Input: part model. Units: mm. Frame: model coordinates. Face numbers are marked on the shaded views. A direction names the side the tool comes from. Round coordinates to 2 decimals unless told otherwise and drop trailing zeros. Loops run counter-clockwise (first coordinate to the right, second up) from the corner with the lowest first, then second, coordinate; pieces in that order, holes last. Notation, with made-up numbers: M 33,16.25 L 81,16.25 A21 cw 81,48.25 Z; hole C -13,9.25 d11. An arc over 180 degrees is marked long. Return JSON: item names as keys, results as strings. Group by question number.
1) Access query for the marked faces 5, 6, 7 and 8. Directions: +Z, -Z, +X, -X, +Y, -Y. A direction counts if a zero-diameter tool reaches every point of the face in a straight line with its end or side. Return the directions, or none.
2) Section C-C (x = 0). Output: boundary loops of the cut face in (y, z).
3) Contact query for flat-ended pins moving along their axis: P1, Ø3.5, axis at x = 11, z = -1, coming from the +Y side; P2, Ø9, axis at x = -3.5, z = -5.5, coming from the +Y side; P3, Ø8, axis at x = 0, y = 0, coming from the -Z side. Output: stop coordinate, or through.
4) Section B-B (z = 3.75). Output: boundary loops of the cut face in (x, y).
5) Section D-D (y = -4.75). Output: boundary loops of the cut face in (x, z), plus the area to 3 significant figures.
6) Mould query, pull axis Y, two halves, no side actions, for the marked faces 1, 2, 3 and 4. Classes: +Y half, -Y half, draft (parallel to the pull), parting line (faces both ways), or undercut.
7) Section A-A (z = -7.75). Output: boundary loops of the cut face in (x, y).
8) Material intervals for line 1 (Y direction, x = 0, z = 2.5); line 2 (X direction, y = -8, z = -2.25); line 3 (X direction, y = 0, z = 4), sorted ascending. Write a range as from..to.
from build123d import *

# Parameters (mm, degrees)
PAD_DEPTH       = 10
SKETCH001_R     = 2.55
POCKET_DEPTH    = 8
CHAMFER_SIZE    = 4
PAD001_DEPTH    = 10
SKETCH003_W     = 13
SKETCH003_H     = 6.844848
POCKET001_DEPTH = 19.501
FILLET_R        = 2


with BuildPart() as part:
    # Sketch → Pad (new body)
    with BuildSketch(Plane.XY):
        Polygon((-4.5, 8.5), (4.5, 8.5), (9, 4), (13.5, 4), (13.5, -11), (-13.5, -11), (-13.5, 4), (-9, 4), align=None)
    extrude(amount=PAD_DEPTH)

    # Sketch001 → Pocket (cut)
    with BuildSketch(Plane(origin=(0, 0, 0), x_dir=(1, 0, 0), z_dir=(0, 0, -1))):
        Circle(SKETCH001_R)
    extrude(amount=-POCKET_DEPTH, mode=Mode.SUBTRACT)

    # Chamfer
    chamfer_edges = [part.edges().sort_by_distance(p)[0] for p in [
        (0, 8.5, 10),
        (6.75, 6.25, 10),
        (11.25, 4, 10),
        (13.5, -3.5, 10),
        (0, -11, 10),
        (-13.5, -3.5, 10),
        (-11.25, 4, 10),
        (-6.75, 6.25, 10),
    ]]
    chamfer(chamfer_edges, length=CHAMFER_SIZE)

    # Sketch002 → Pad001 (new body)
    with BuildSketch(Plane(origin=(0, 0, 0), x_dir=(1, 0, 0), z_dir=(0, 0, -1))):
        Polygon((-13.5, -4), (-12.5, -4), (-12.5, 10), (12.5, 10), (12.5, -4), (13.5, -4), (13.5, 11), (-13.5, 11), align=None)
    extrude(amount=PAD001_DEPTH)

    # Sketch003 → Pocket001 (cut, through all)
    with BuildSketch(Plane.XZ.offset(11)):
        with Locations((0, -8.422424)):
            Rectangle(SKETCH003_W, SKETCH003_H)
    extrude(amount=-POCKET001_DEPTH, mode=Mode.SUBTRACT)

    # Fillet
    fillet_edges = [part.edges().sort_by_distance(p)[0] for p in [
        (12.5, -3, 0),
        (0, -10, 0),
        (-12.5, -3, 0),
    ]]
    fillet(fillet_edges, radius=FILLET_R)


solid = part.part
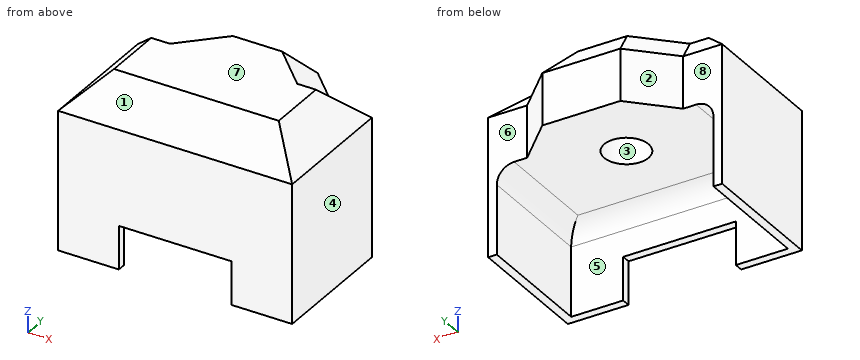
Returned:
{
 "1": {"face 5": "-Z, +Y", "face 6": "+Z, -Z, +X, +Y", "face 7": "+Z, +X, -X, +Y, -Y", "face 8": "+Z, -Z, -X, +Y"},
 "2": {"outline": "M -11,-5 L -10,-5 L -10,-2 A2 cw -8,0 L -2.55,0 L -2.55,8 L 2.55,8 L 2.55,0 L 8.5,0 L 8.5,6 L 4.5,10 L -7,10 L -11,6 Z"},
 "3": {"P1": "stops at y = 4", "P2": "stops at y = -9.73", "P3": "stops at z = 0"},
 "4": {"outline": "M -13.5,-11 L 13.5,-11 L 13.5,4 L 9,4 L 4.5,8.5 L -4.5,8.5 L -9,4 L -13.5,4 Z; hole C 0,0 d5.1"},
 "5": {"outline": "M -13.5,-10 L -12.5,-10 L -12.5,-2 A2 cw -10.5,0 L 10.5,0 A2 cw 12.5,-2 L 12.5,-10 L 13.5,-10 L 13.5,6 L 9.5,10 L -9.5,10 L -13.5,6 Z", "area": "276 mm^2"},
 "6": {"face 1": "-Y half", "face 2": "+Y half", "face 3": "undercut", "face 4": "draft"},
 "7": {"outline": "M -13.5,-11 L -6.5,-11 L -6.5,-10 L -12.5,-10 L -12.5,4 L -13.5,4 Z; M 6.5,-11 L 13.5,-11 L 13.5,4 L 12.5,4 L 12.5,-10 L 6.5,-10 Z"},
 "8": {"line 1": "y = -11..-2.55, 2.55..8.5", "line 2": "x = -13.5..-12.5, 12.5..13.5", "line 3": "x = -13.5..-2.55, 2.55..13.5"}
}
